Could you check a few things on this model? Use its own coordinates, in mm. Give positions to 0.01 mm unless a question says otherwise; leave off trailing zeros. Loops run counter-clockwise (first coordinate to the right, second up) from the corner with the lowest first, then second, coordinate; pieces in that order, holes last. Notation, with made-up numbers: M 54.5,8.25 L 100.5,8.25 A29 cw 100.5,28.25 Z; hole C -38.5,-13.75 d10. An arc over 180 degrees is marked long. Return JSON: item names as keys, results as strings. Group by question number.
1. If we section it at B-B (y = 3.5): State how many separate pieces and enclosed holes the cut face has, plus the area to 3 significant figures.
2. Please list where these lines run through material, in increasing order: line 1 (X direction, y = 2, z = 17); line 2 (X direction, y = -5, z = 4.5); line 3 (Y direction, x = 68.5, z = 18.25).
3. For pin 1 (2 mm diameter, centred on y = -26.5, z = 9.5, fed in from +X); pin 2 (6 mm diameter, centred on x = 3, y = -9.5, fed in from -Z); pin 3 (3 mm diameter, centred on y = -18.5, z = 12.5, fed in from -X); pin 4 (8 mm diameter, centred on y = 25.5, z = 8, fed in from -X), each with a flat end and sliding along its axis, tell me the tip position at first contact or that it passes through.
4. If we section it at A-A (z = 3.75): Write out the boundary of the cut face in (x, y), plus the area to 3 significant figures.
```python
from build123d import *

# Parameters (mm, degrees)
F1_DEPTH = 25.4
F2_SIZE  = 5.08
F3_R     = 5.08


with BuildPart() as f1:
    # F0 (on Top) → F1 (new body)
    with BuildSketch(Plane.XY):
        with BuildLine():
            Line((-70.3059094878, 6.35), (-70.3059094878, 38.1))
            Line((-70.3059094878, 38.1), (-114.3, -38.1))
            Line((-114.3, -38.1), (-70.3059094878, -38.1))
            Line((-70.3059094878, -38.1), (-70.3059094878, -6.35))
            ThreePointArc((-70.3059094878, -6.35), (-76.6559094878, 0), (-70.3059094878, 6.35))
        make_face()
        with BuildLine():
            Line((70.3059094878, 6.35), (70.3059094878, 38.1))
            Line((70.3059094878, 38.1), (-70.3059094878, 38.1))
            Line((-70.3059094878, 38.1), (-70.3059094878, 6.35))
            ThreePointArc((-70.3059094878, 6.35), (-65.8157814272, 4.4901280605), (-63.9559094878, 0))
            ThreePointArc((-63.9559094878, 0), (-65.8157814272, -4.4901280605), (-70.3059094878, -6.35))
            Line((-70.3059094878, -6.35), (-70.3059094878, -38.1))
            Line((-70.3059094878, -38.1), (70.3059094878, -38.1))
            Line((70.3059094878, -38.1), (70.3059094878, -6.35))
            ThreePointArc((70.3059094878, -6.35), (63.9559094878, 0), (70.3059094878, 6.35))
        make_face()
        with BuildLine():
            Line((114.3, -38.1), (70.3059094878, 38.1))
            Line((70.3059094878, 38.1), (70.3059094878, 6.35))
            ThreePointArc((70.3059094878, 6.35), (74.7960375483, 4.4901280605), (76.6559094878, 0))
            ThreePointArc((76.6559094878, 0), (74.7960375483, -4.4901280605), (70.3059094878, -6.35))
            Line((70.3059094878, -6.35), (70.3059094878, -38.1))
            Line((70.3059094878, -38.1), (114.3, -38.1))
        make_face()
    extrude(amount=F1_DEPTH)

    # F2
    f2_edges = [f1.edges().sort_by_distance(p)[0] for p in [
        (-70.305909, -6.35, 25.4),
        (70.305909, -6.35, 25.4),
    ]]
    chamfer(f2_edges, length=F2_SIZE)

    # F3
    f3_edges = [f1.edges().sort_by_distance(p)[0] for p in [
        (0, -38.1, 25.4),
        (-92.302955, 0, 25.4),
        (0, 38.1, 25.4),
        (92.302955, 0, 25.4),
    ]]
    fillet(f3_edges, radius=F3_R)


solid = f1.part
```
Answer:
{
 "1": {"separate pieces": "3", "enclosed holes": "0", "area": "3,980 mm²"},
 "2": {"line 1": "x = -91.15 to -76.33, -64.28 to 64.28, 76.33 to 91.15", "line 2": "x = -95.19 to -74.22, -66.39 to 66.39, 74.22 to 95.19", "line 3": "y = -38.1 to -6.09, 6.09 to 38.1"},
 "3": {"pin 1": "stops at x = 108.18", "pin 2": "stops at z = 0", "pin 3": "stops at x = -103.85", "pin 4": "stops at x = -79.89"},
 "4": {"outline": "M -114.3,-38.1 L 114.3,-38.1 L 70.31,38.1 L -70.31,38.1 Z; hole C -70.31,0 d12.7; hole C 70.31,0 d12.7", "area": "13,800 mm²"}
}
